Geometry check sheet. Reference: drawing and pictorial views, mm from the part's lowest x, y, z. Coordinates: 2 decimals unless noted, no trailing zeros. Loops run counter-clockwise (first coordinate to the right, second up) from the corner with the lowest first, then second, coordinate; pieces in that order, holes last.
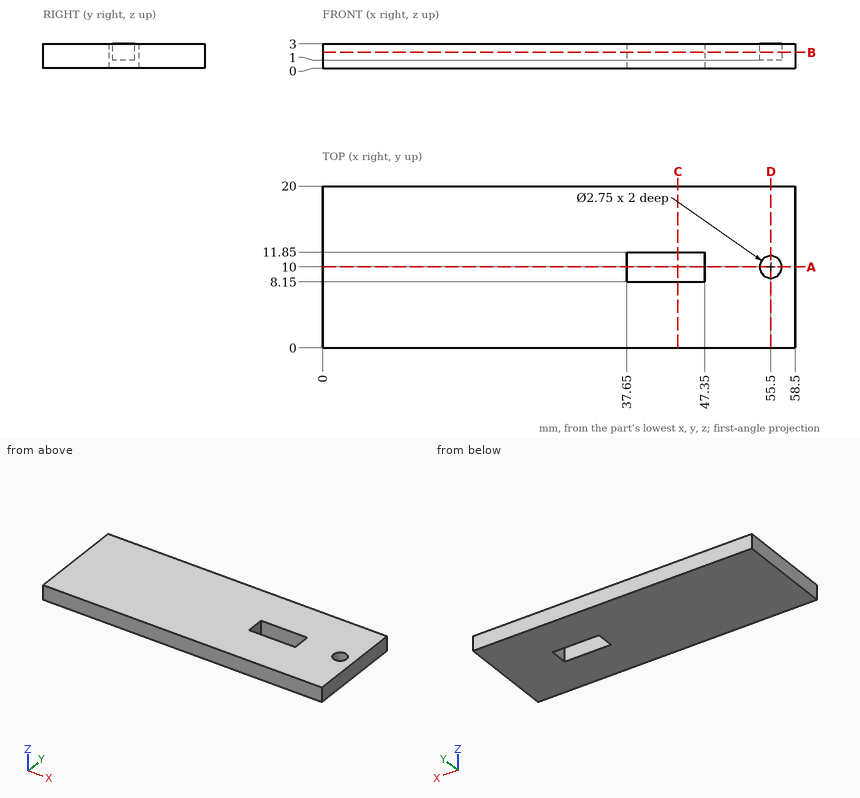
1) Section check C-C on x = 44. Record the cut outline in (y, z), and give its area (3 significant figures).
Data:
outline: (0, 0) - (8.15, 0) - (8.15, 3) - (0, 3) - close; (11.85, 0) - (20, 0) - (20, 3) - (11.85, 3) - close
area: 48.9 mm2
2) Section check B-B on z = 1.95. Record the cut outline in (x, y) (3 decimals), and give its area (3 significant figures).
Data:
outline: (0, 0) - (58.5, 0) - (58.5, 20) - (0, 20) - close; hole (37.65, 8.15) - (47.35, 8.15) - (47.35, 11.85) - (37.65, 11.85) - close; hole circle Ø2.75 at (55.5, 10)
area: 1,130 mm2
3) Section check A-A on y = 10. Record the cut outline in (x, z) (3 decimals).
Data:
outline: (0, 0) - (37.65, 0) - (37.65, 3) - (0, 3) - close; (47.35, 0) - (58.5, 0) - (58.5, 3) - (56.875, 3) - (56.875, 1) - (54.125, 1) - (54.125, 3) - (47.35, 3) - close
4) Section check D-D on x = 55.5. Record the cut outline in (y, z) (3 decimals).
Data:
outline: (0, 0) - (20, 0) - (20, 3) - (11.375, 3) - (11.375, 1) - (8.625, 1) - (8.625, 3) - (0, 3) - close
5) Depth check by flat-ended pin: pin 1 (0.8 mm diameter, centred on x = 55, y = 10.5, fed in from +Z). Enter the tip coordinate at first touch or a pass-through.
Data:
pin 1: stops at z = 1
6) Material ranges on probe 1 along Y at (x, z) = (45, 2.85); probe 2 along Y at (x, z) = (55.5, 1.8) (3 decimals); probe 3 along X at (y, z) = (10.75, 2.4), recorded low to high.
Data:
probe 1: y = 0 to 8.15, 11.85 to 20
probe 2: y = 0 to 8.625, 11.375 to 20
probe 3: x = 0 to 37.65, 47.35 to 54.35, 56.65 to 58.5
